```python
from build123d import *

# Parameters (mm, degrees)
SKETCH1_W                = 127.979014886
SKETCH1_H                = 127.125142163
BOSS_EXTRUDE1_DEPTH      = 2.286
SKETCH2_W                = 127.979014886
SKETCH2_H                = 127.125142163
BOSS_EXTRUDE2_DEPTH      = 76.2
SKETCH4_W                = 123.407014886
SKETCH4_H                = 122.553142163
CUT_EXTRUDE2_DEPTH       = 76.2
SKETCH5_W                = 123.407014886
SKETCH5_H                = 76.2
CUT_EXTRUDE3_DEPTH       = 2.286
SKETCH6_W                = 123.407014886
SKETCH6_H                = 65.786
CUT_EXTRUDE4_DEPTH       = 2.286
SKETCH7_W                = 127.125142163
SKETCH7_H                = 38.112983868
CUT_EXTRUDE5_DEPTH       = 2.286
SKETCH8_W                = 31.75
SKETCH8_H                = 2.854777597
CUT_EXTRUDE6_DEPTH       = 2.54
SKETCH9_W                = 2.286
SKETCH9_H                = 4.572
BOSS_EXTRUDE3_DEPTH      = 76.2
SKETCH11_W               = 2.286
SKETCH11_H               = 4.572
BOSS_EXTRUDE5_DEPTH      = 38.1
BOSS_EXTRUDE6_DEPTH      = 27.686
BOSS_EXTRUDE6_DEPTH_BACK = 10.414
SKETCH12_W               = 2.286
SKETCH12_H               = 4.697142163
BOSS_EXTRUDE7_DEPTH      = 65.786
BOSS_EXTRUDE7_DEPTH_BACK = 10.414
SKETCH13_W               = 2.286
SKETCH13_H               = 4.572
SKETCH14_R               = 1.524
CUT_EXTRUDE7_DEPTH       = 6.35
SKETCH15_R               = 1.524
CUT_EXTRUDE8_DEPTH       = 6.35
SKETCH16_R               = 1.524
CUT_EXTRUDE9_DEPTH       = 6.35
SKETCH18_R               = 1.524
CUT_EXTRUDE10_DEPTH      = 6.35
SKETCH19_R               = 1.524
CUT_EXTRUDE11_DEPTH      = 6.35
FILLET1_R                = 1.27
FILLET2_R                = 1.27
FILLET7_R                = 1.27
FILLET8_R                = 1.27


with BuildPart() as part:
    # Sketch1 → Boss-Extrude1 (new body)
    with BuildSketch(Plane(origin=(0, 0, 0), x_dir=(1, 0, 0), z_dir=(0, 1, 0))):
        with Locations((63.989507443, 63.562571082)):
            Rectangle(SKETCH1_W, SKETCH1_H)
    extrude(amount=BOSS_EXTRUDE1_DEPTH)

    # Sketch2 → Boss-Extrude2 (add)
    with BuildSketch(Plane(origin=(0, 2.286, 0), x_dir=(1, 0, 0), z_dir=(0, 1, 0))):
        with Locations((63.989507443, 63.562571082)):
            Rectangle(SKETCH2_W, SKETCH2_H)
    extrude(amount=BOSS_EXTRUDE2_DEPTH)

    # Sketch4 → Cut-Extrude2 (cut)
    with BuildSketch(Plane(origin=(0, 78.486, 0), x_dir=(1, 0, 0), z_dir=(0, 1, 0))):
        with Locations((63.989507443, 63.562571082)):
            Rectangle(SKETCH4_W, SKETCH4_H)
    extrude(amount=-CUT_EXTRUDE2_DEPTH, mode=Mode.SUBTRACT)

    # Sketch5 → Cut-Extrude3 (cut)
    with BuildSketch(Plane.XY):
        with Locations((63.989507443, 40.386)):
            Rectangle(SKETCH5_W, SKETCH5_H)
    extrude(amount=-CUT_EXTRUDE3_DEPTH, mode=Mode.SUBTRACT)

    # Sketch6 → Cut-Extrude4 (cut)
    with BuildSketch(Plane(origin=(0, 0, -127.125142163), x_dir=(-1, 0, 0), z_dir=(0, 0, -1))):
        with Locations((-63.989507443, 45.593)):
            Rectangle(SKETCH6_W, SKETCH6_H)
    extrude(amount=-CUT_EXTRUDE4_DEPTH, mode=Mode.SUBTRACT)

    # Sketch7 → Cut-Extrude5 (cut)
    with BuildSketch(Plane.ZY):
        with Locations((-63.562571082, 59.429508066)):
            Rectangle(SKETCH7_W, SKETCH7_H)
    extrude(amount=-CUT_EXTRUDE5_DEPTH, mode=Mode.SUBTRACT)

    # Sketch8 → Cut-Extrude6 (cut)
    with BuildSketch(Plane.ZY):
        with Locations((-79.500142163, 38.945627333)):
            Rectangle(SKETCH8_W, SKETCH8_H)
    extrude(amount=-CUT_EXTRUDE6_DEPTH, mode=Mode.SUBTRACT)

    # Sketch9 → Boss-Extrude3 (add)
    with BuildSketch(Plane(origin=(0, 2.286, 0), x_dir=(1, 0, 0), z_dir=(0, 1, 0))):
        with Locations((124.550014886, 2.286)):
            Rectangle(SKETCH9_W, SKETCH9_H)
    extrude(amount=BOSS_EXTRUDE3_DEPTH)

    # Sketch11 → Boss-Extrude5 (add)
    with BuildSketch(Plane(origin=(0, 2.286, 0), x_dir=(1, 0, 0), z_dir=(0, 1, 0))):
        with Locations((3.429, 2.286)):
            Rectangle(SKETCH11_W, SKETCH11_H)
    extrude(amount=BOSS_EXTRUDE5_DEPTH)

    # Sketch12 → Boss-Extrude6 (add, two sides: drawn at the far end of the back side and taken through both)
    with BuildSketch(Plane(origin=(0, 12.7, 0), x_dir=(1, 0, 0), z_dir=(0, 1, 0)).offset(-BOSS_EXTRUDE6_DEPTH_BACK)):
        with Locations((3.429, 124.776571082)):
            Rectangle(SKETCH12_W, SKETCH12_H)
    extrude(amount=BOSS_EXTRUDE6_DEPTH + BOSS_EXTRUDE6_DEPTH_BACK)

    # Sketch13 → Boss-Extrude7 (add, two sides: drawn at the far end of the back side and taken through both)
    with BuildSketch(Plane(origin=(0, 12.7, 0), x_dir=(1, 0, 0), z_dir=(0, 1, 0)).offset(-BOSS_EXTRUDE7_DEPTH_BACK)):
        with Locations((124.550014886, 124.839142163)):
            Rectangle(SKETCH13_W, SKETCH13_H)
    extrude(amount=BOSS_EXTRUDE7_DEPTH + BOSS_EXTRUDE7_DEPTH_BACK)

    # Sketch14 → Cut-Extrude7 (cut)
    with BuildSketch(Plane(origin=(0, 78.486, 0), x_dir=(1, 0, 0), z_dir=(0, 1, 0))):
        with Locations(Location((125.693014886, 2.286, 0), (0, 0, 270))):
            Circle(SKETCH14_R)
    extrude(amount=-CUT_EXTRUDE7_DEPTH, mode=Mode.SUBTRACT)

    # Sketch15 → Cut-Extrude8 (cut)
    with BuildSketch(Plane(origin=(0, 78.486, 0), x_dir=(1, 0, 0), z_dir=(0, 1, 0))):
        with Locations(Location((125.693014886, 124.839142163, 0), (0, 0, 270))):
            Circle(SKETCH15_R)
    extrude(amount=-CUT_EXTRUDE8_DEPTH, mode=Mode.SUBTRACT)

    # Sketch16 → Cut-Extrude9 (cut)
    with BuildSketch(Plane(origin=(0, 40.373016132, 0), x_dir=(1, 0, 0), z_dir=(0, 1, 0))):
        with Locations(Location((2.286, 2.286, 0), (0, 0, 270))):
            Circle(SKETCH16_R)
    extrude(amount=-CUT_EXTRUDE9_DEPTH, mode=Mode.SUBTRACT)

    # Sketch18 → Cut-Extrude10 (cut)
    with BuildSketch(Plane(origin=(0, 40.386, 0), x_dir=(1, 0, 0), z_dir=(0, 1, 0))):
        with Locations(Location((2.286, 2.286, 0), (0, 0, 270))):
            Circle(SKETCH18_R)
    extrude(amount=-CUT_EXTRUDE10_DEPTH, mode=Mode.SUBTRACT)

    # Sketch19 → Cut-Extrude11 (cut)
    with BuildSketch(Plane(origin=(0, 40.386, 0), x_dir=(1, 0, 0), z_dir=(0, 1, 0))):
        with Locations(Location((2.286, 124.776571082, 0), (0, 0, 270))):
            Circle(SKETCH19_R)
    extrude(amount=-CUT_EXTRUDE11_DEPTH, mode=Mode.SUBTRACT)

    # Fillet1
    fillet1_edges = [part.edges().sort_by_distance(p)[0] for p in [
        (0, 20.186508066, 0),
    ]]
    fillet(fillet1_edges, radius=FILLET1_R)

    # Fillet2
    fillet2_edges = [part.edges().sort_by_distance(p)[0] for p in [
        (4.572, 21.336, 0),
        (4.572, 21.336, -4.572),
        (4.572, 26.543, -127.125142163),
        (63.989507443, 12.7, -127.125142163),
        (123.407014886, 45.593, -127.125142163),
        (64.624507443, 0, 0),
        (0, 0, -64.197571082),
        (0.371974388, 0, -0.371974388),
        (127.979014886, 0, -63.562571082),
        (63.989507443, 0, -127.125142163),
        (0, 20.186508066, -127.125142163),
        (127.979014886, 39.243, -127.125142163),
    ]]
    fillet(fillet2_edges, radius=FILLET2_R)

    # Fillet7
    fillet7_edges = [part.edges().sort_by_distance(p)[0] for p in [
        (4.572, 21.336, -122.428),
    ]]
    fillet(fillet7_edges, radius=FILLET7_R)

    # Fillet8
    # the kernel refuses this fillet: 1.27 mm, written as the material it takes off along each edge
    with BuildSketch(Plane(origin=(126.709014886, 1.27, -1.27), x_dir=(1, 0, 0), z_dir=(0, 0, 1))) as fillet8_piece_1_section:
        Polygon((0, 0), (FILLET8_R, 0), (FILLET8_R, -FILLET8_R), (0, -FILLET8_R), align=None)
    fillet8_piece_1 = extrude(amount=FILLET8_R, mode=Mode.PRIVATE)
    fillet8_piece_1 = fillet8_piece_1 - Plane(origin=(126.709014886, 1.27, -1.27), x_dir=(-0.7071067811865475, 0.7071067811865475, 0), z_dir=(0, 0, 1)) * Sphere(FILLET8_R, mode=Mode.PRIVATE)
    add(fillet8_piece_1, mode=Mode.SUBTRACT)
    with BuildSketch(Plane(origin=(123.407014886, 2.286, -4.572), x_dir=(1, 0, 0), z_dir=(0, 1, 0)), Plane(origin=(123.407014886, 2.286, 0), x_dir=(0, 0, -1), z_dir=(0, 1, 0)), Plane(origin=(123.407014886, 2.286, -122.553142163), x_dir=(0, 0, -1), z_dir=(0, 1, 0))) as fillet8_piece_2:
        with BuildLine():
            CenterArc((FILLET8_R, -FILLET8_R), FILLET8_R, 90, 90)
            Line((0, -FILLET8_R), (0, 0))
            Line((0, 0), (FILLET8_R, 0))
        make_face()
    extrude(amount=79.375, mode=Mode.SUBTRACT)
    with BuildSketch(Plane(origin=(127.979014886, 1.27, 0), x_dir=(-1, 0, 0), z_dir=(0, 1, 0))) as fillet8_piece_3:
        with BuildLine():
            CenterArc((FILLET8_R, -FILLET8_R), FILLET8_R, 90, 90)
            Line((0, -FILLET8_R), (0, 0))
            Line((0, 0), (FILLET8_R, 0))
        make_face()
    extrude(amount=80.391, mode=Mode.SUBTRACT)


solid = part.part
```
CAD build for the part. Positions are in the model's coordinates, mm. A direction names the side the tool comes from. Coordinates: 2 decimals unless noted, no trailing zeros. Order: outer loops, then holes, each group sorted by start corner. A loop starts at its lowest first (then second) coordinate and runs counter-clockwise, first axis right, second up. Notation, with made-up numbers: (42, 19) - (89, 19) arc R18 cw to (89, 24) - close; hole circle Ø8 at (69, -32.5). An arc over 180 degrees is marked (long way). Use a Markdown table: item, result. Add a question column.
(1) Drill centre lines: line 1 along X through (y, z) = (28, -32.5); line 2 along Y through (x, z) = (23.5, -101.5); line 3 along X through (y, z) = (64.5, -109). Where is each one in solid material? Low to high. Write a range as [from, to].
(2) Saw through at D-D (y = 6.5). Give the cut face in (x, z), then the cut area to 3 significant figures.
(3) Saw through at A-A (y = 24). Give the cut face in (x, z), then the cut area to 3 significant figures.
(4) Which spindle directions (+Z, -Z, +X, -X, +Y, -Y) get a long thin tool onto all of the face, cutting with end or side? Do faces 4 (the face through (63, 8, -124.839)), 5 (the face through (127.979, 39, -63)), 6 (the face through (125.693, 40, -64)). Say none if no direction does.
(5) Pull direction Z, two halves, no side cores. Call faces 1 (the face through (0, 21, -63)), 2 (the face through (126, 72.136, -125)), 3 (the face through (3, 23, 0)): +Z half, -Z half, draft (parallel to the pull), parting line (faces both ways), or undercut.
(6) Saw through at B-B (z = -53). Give the cut face in (x, y).
(7) Saw through at C-C (x = 48). Give the cut face in (y, z).
(8) Flat gauge pins, fed straight in: pin 1 (5 mm diameter, centred on x = 68.5, y = 5, fed in from +Z); pin 2 (0.7 mm diameter, centred on x = 1, z = -75, fed in from +Y); pin 3 (10 mm diameter, centred on x = 80, z = -43.5, fed in from +Y). Where does each tip first touch, or does it go through?
Solved:
| question | item | result |
|---|---|---|
| 1 | line 1 | x = [0, 2.29], [125.69, 127.98] |
| 1 | line 2 | y = [0, 2.29] |
| 1 | line 3 | x = [125.69, 127.98] |
| 2 | outline | (0, -125.86) arc R1.27 ccw to (1.27, -127.13) - (126.71, -127.13) arc R1.27 ccw to (127.98, -125.86) - (127.98, -1.27) arc R1.27 ccw to (126.71, 0) - (124.68, 0) arc R1.27 ccw to (123.41, -1.27) - (123.41, -3.3) arc R1.27 ccw to (124.68, -4.57) - (125.69, -4.57) - (125.69, -122.55) - (124.68, -122.55) arc R1.27 ccw to (123.41, -123.82) - (123.41, -124.84) - (4.57, -124.84) - (4.57, -123.7) arc R1.27 ccw to (3.3, -122.43) - (2.29, -122.43) - (2.29, -4.57) - (3.3, -4.57) arc R1.27 ccw to (4.57, -3.3) - (4.57, -1.27) arc R1.27 ccw to (3.3, 0) - (1.27, 0) arc R1.27 ccw to (0, -1.27) - close |
| 2 | area | 892 mm² |
| 3 | outline | (0, -125.86) arc R1.27 ccw to (1.27, -127.13) - (3.3, -127.13) arc R1.27 ccw to (4.57, -125.86) - (4.57, -123.7) arc R1.27 ccw to (3.3, -122.43) - (2.29, -122.43) - (2.29, -4.57) - (3.3, -4.57) arc R1.27 ccw to (4.57, -3.3) - (4.57, -1.27) arc R1.27 ccw to (3.3, 0) - (1.27, 0) arc R1.27 ccw to (0, -1.27) - close; (123.41, -125.86) arc R1.27 ccw to (124.68, -127.13) - (126.71, -127.13) arc R1.27 ccw to (127.98, -125.86) - (127.98, -1.27) arc R1.27 ccw to (126.71, 0) - (124.68, 0) arc R1.27 ccw to (123.41, -1.27) - (123.41, -3.3) arc R1.27 ccw to (124.68, -4.57) - (125.69, -4.57) - (125.69, -122.55) - (124.68, -122.55) arc R1.27 ccw to (123.41, -123.82) - close |
| 3 | area | 619 mm² |
| 4 | face 4 | +Z, +Y |
| 4 | face 5 | +Z, -Z, +X, +Y, -Y |
| 4 | face 6 | +Y |
| 5 | face 1 | draft |
| 5 | face 2 | undercut |
| 5 | face 3 | +Z half |
| 6 | outline | (0, 1.27) arc R1.27 ccw to (1.27, 0) - (126.71, 0) arc R1.27 ccw to (127.98, 1.27) - (127.98, 78.49) - (125.69, 78.49) - (125.69, 2.29) - (2.29, 2.29) - (2.29, 40.37) - (0, 40.37) - close |
| 7 | outline | (0, -125.86) arc R1.27 ccw to (1.27, -127.13) - (11.43, -127.13) arc R1.27 ccw to (12.7, -125.86) - (12.7, -124.84) - (2.29, -124.84) - (2.29, 0) - (1.27, 0) arc R1.27 ccw to (0, -1.27) - close |
| 8 | pin 1 | stops at z = -124.84 |
| 8 | pin 2 | stops at y = 37.52 |
| 8 | pin 3 | stops at y = 2.29 |
